Model file for the job. Use its own axes, mm. A direction names the side the tool comes from. Round coordinates to 2 decimals unless told otherwise and drop trailing zeros. Loops run counter-clockwise (first coordinate to the right, second up) from the corner with the lowest first, then second, coordinate; pieces in that order, holes last. Notation, with made-up numbers: (20, 1.25) -> (70, 1.25) arc R16 cw to (70, 12.25) -> close; hole circle Ø2 at (82, -28). An arc over 180 degrees is marked (long way). Use a Markdown table: item, result.
from build123d import *

# Parameters (mm, degrees)
ESBO_O1_R                = 1.5
RESSALTO_EXTRUS_O1_DEPTH = 3


with BuildPart() as part:
    # Esboço1 → Ressalto-extrusão1 (new body)
    with BuildSketch(Plane(origin=(0, 0, 0), x_dir=(1, 0, 0), z_dir=(0, 1, 0))):
        Polygon((6.5, 16.127416998), (6.5, 45), (-6.5, 45), (-6.5, 16.127416998), (-16.127416998, 6.5), (-45, 6.5), (-45, -6.5), (-16.127416998, -6.5), (0, -22.627416998), (16.127416998, -6.5), (45, -6.5), (45, 6.5), (16.127416998, 6.5), align=None)
        with Locations(Location((0, -12, 0), (0, 0, 270))):
            Circle(ESBO_O1_R, mode=Mode.SUBTRACT)
        with Locations(Location((0, 12, 0), (0, 0, 270))):
            Circle(ESBO_O1_R, mode=Mode.SUBTRACT)
    extrude(amount=RESSALTO_EXTRUS_O1_DEPTH)


solid = part.part
Q1. Band-saw the part on A-A, the plane y = 2.3. Give the cut face in (x, z), plus the area to 3 significant figures.
Results list:
| item | result |
|---|---|
| outline | (-45, -6.5) -> (-16.13, -6.5) -> (-6.5, -16.13) -> (-6.5, -45) -> (6.5, -45) -> (6.5, -16.13) -> (16.13, -6.5) -> (45, -6.5) -> (45, 6.5) -> (16.13, 6.5) -> (0, 22.63) -> (-16.13, 6.5) -> (-45, 6.5) -> close; hole circle Ø3 at (0, -12); hole circle Ø3 at (0, 12) |
| area | 2,010 mm² |
Q2. Pull direction X, two halves, no side cores. Call faces 1 (the face through (0.07, 1.48, -13.5)), 2 (the face through (31, 1, -6.5)), 3 (the face through (-11.25, 1.48, -11.38)): released by +X, released by -X, zero draft, split by the parting line, or undercut.
Results list:
| item | result |
|---|---|
| face 1 | undercut |
| face 2 | zero draft |
| face 3 | released by -X |
Q3. Band-saw the part on D-D, the plane z = -25. Give the cut face in (x, y).
Results list:
| item | result |
|---|---|
| outline | (-6.5, 0) -> (6.5, 0) -> (6.5, 3) -> (-6.5, 3) -> close |
Q4. Band-saw the part on B-B, the plane z = -12. Give the cut face in (x, y), plus the area to 3 significant figures.
Results list:
| item | result |
|---|---|
| outline | (-10.63, 0) -> (-1.5, 0) -> (-1.5, 3) -> (-10.63, 3) -> close; (1.5, 0) -> (10.63, 0) -> (10.63, 3) -> (1.5, 3) -> close |
| area | 54.8 mm² |
Q5. Tool access for faces 4 (the face through (30, 1, 6.5)), 5 (the face through (-31, 1, 6.5)), 6 (the face through (6.5, 1, -30)), 7 (the face through (-6.5, 1, -31)): list every direction of +Z, -Z, +X, -X, +Y, -Y with a clear straight run to the whole face (end or side of a thin tool).
Results list:
| item | result |
|---|---|
| face 4 | +Z, +X, +Y, -Y |
| face 5 | +Z, -X, +Y, -Y |
| face 6 | -Z, +X, +Y, -Y |
| face 7 | -Z, -X, +Y, -Y |
Q6. Drill centre lines: L1, parallel to Z at x = -28, y = 1.3; L2, parallel to X at y = 2.8, z = -12.5. Where is each one in solid material? Low to high. Write a range as from..to.
Results list:
| item | result |
|---|---|
| L1 | z = -6.5..6.5 |
| L2 | x = -10.13..-1.41, 1.41..10.13 |
Q7. Flat gauge pins, fed straight in: pin 1 (0.9 mm diameter, centred on x = 36.5, y = 1.5, fed in from -Z); pin 2 (1 mm diameter, centred on y = 0.5, z = -22, fed in from -X); pin 3 (1.5 mm diameter, centred on y = 1, z = -32, fed in from +X). Where does each tip first touch, or does it go through?
Results list:
| item | result |
|---|---|
| pin 1 | stops at z = -6.5 |
| pin 2 | stops at x = -6.5 |
| pin 3 | stops at x = 6.5 |
Q8. Band-saw the part on C-C, the plane x = 37.5. Give the cut face in (y, z).
Results list:
| item | result |
|---|---|
| outline | (0, -6.5) -> (3, -6.5) -> (3, 6.5) -> (0, 6.5) -> close |
